Answer from the drawing. Dimensions are ordinates in mm from the lowest x, y and z of the part. Give positions to 0.01 mm unless a question says otherwise; leave off trailing zeros. Loops run counter-clockwise (first coordinate to the right, second up) from the corner with the lowest first, then second, coordinate; pieces in that order, holes last.
(1) Find section A-A, the plane x = 4.5. Write down the section's boundary in (y, z).
(2) Find section B-B, the plane z = 28. Write down the section's boundary in (x, y), then the cut area to 3 significant figures.
(3) Each of these flat-tipped pins is pushed along its axis until it touches: P1, Ø3, axis at x = 16.5, y = 7, coming from the +Z side; P2, Ø5, axis at x = 11.5, y = 42, coming from the +Z side; P3, Ø2, axis at x = 21, y = 8.5, coming from the +Z side (1 decimal). Where does it stop, or does it pass through?
(4) Straight lines are drawn through the part: probe 1 along X at (y, z) = (36.5, 18.5); probe 2 along X at (y, z) = (21, 17); probe 3 along Z at (x, y) = (40.5, 10.5) (1 decimal). For each, find the intervals that lie inside material, in ascending order.
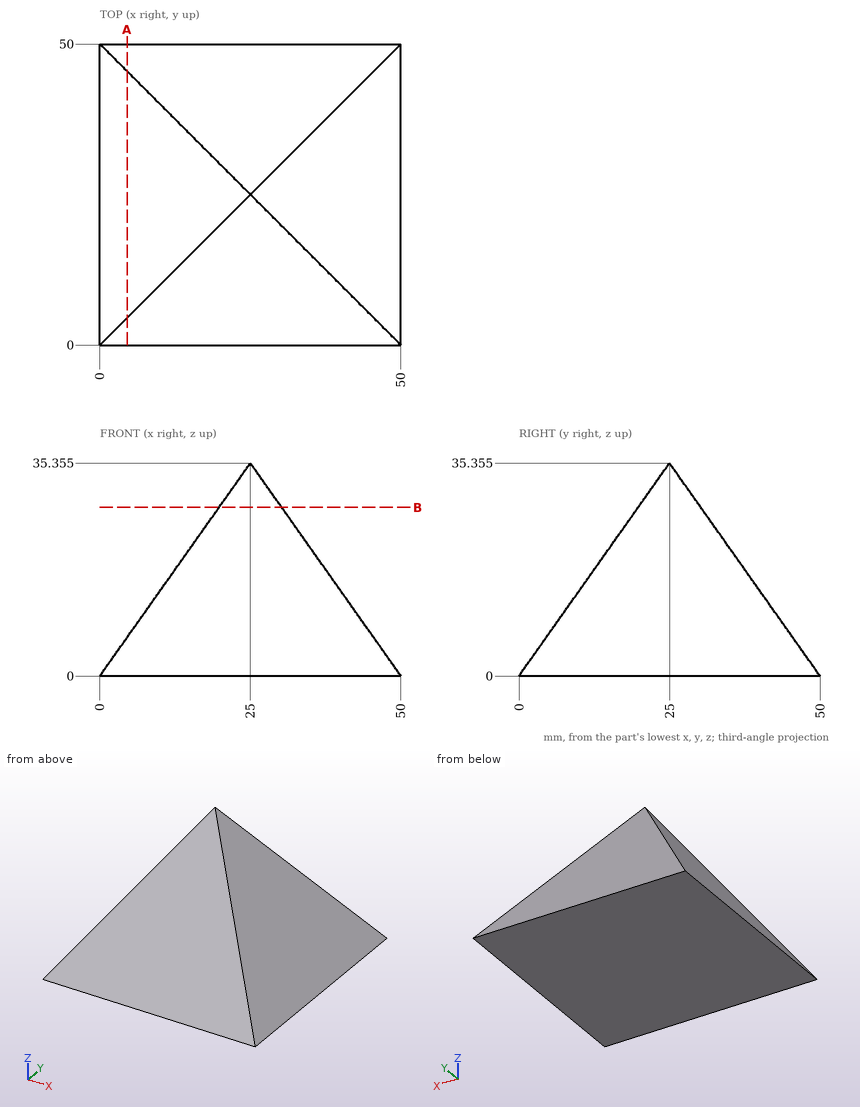
Entries:
1. outline: (0, 0) - (50, 0) - (45.5, 6.36) - (4.5, 6.36) - close
2. outline: (19.8, 19.8) - (30.2, 19.8) - (30.2, 30.2) - (19.8, 30.2) - close
2. area: 108 mm2
3. P1: stops at z = 12.02
3. P2: stops at z = 14.85
3. P3: stops at z = 13.4
4. probe 1: x = 13.08 to 36.92
4. probe 2: x = 12.02 to 37.98
4. probe 3: z = 0 to 13.4
